from build123d import *

# Parameters (mm, degrees)
EXTRUDE_1_DEPTH     = 16
SKETCH_2_W          = 18.798290213
SKETCH_2_H          = 18.208539932
SKETCH_2_R          = 8
CUT_EXTRUDE_1_DEPTH = 16


with BuildPart() as part:
    # 草图1 → 凸台-拉伸1 (new body)
    with BuildSketch(Plane.XY):
        with BuildLine():
            Line((-8, 0), (-8, 16))
            Line((-8, 16), (8, 16))
            Line((8, 16), (8, 0))
            ThreePointArc((8, 0), (0, -8), (-8, 0))
        make_face()
    extrude(amount=EXTRUDE_1_DEPTH)

    # 草图2 → 切除-拉伸1 (cut)
    with BuildSketch(Plane(origin=(0, 16, 0), x_dir=(1, 0, 0), z_dir=(0, 1, 0))):
        with Locations((-0.294875141, -7.797273341)):
            Rectangle(SKETCH_2_W, SKETCH_2_H)
        with Locations((0, -8)):
            Circle(SKETCH_2_R, mode=Mode.SUBTRACT)
    extrude(amount=-CUT_EXTRUDE_1_DEPTH, mode=Mode.SUBTRACT)


solid = part.part
Geometry check sheet. Reference: the model listing, model coordinates, mm. A direction names the side the tool comes from. Round coordinates to 2 decimals unless told otherwise and drop trailing zeros. Loops run counter-clockwise (first coordinate to the right, second up) from the corner with the lowest first, then second, coordinate; pieces in that order, holes last.
Item 1: Cross-section at A-A on x = 1.5. Record the boundary of the cut face in (y, z), then the cut area to 3 significant figures.
Item 2: Cross-section at B-B on z = 15. Record the boundary of the cut face in (x, y), then the cut area to 3 significant figures.
Item 3: Thickness scan on line 1 (X direction, y = 11.25, z = 7.75); line 2 (X direction, y = -1, z = 14.5); line 3 (Y direction, x = -1.75, z = 10.5). Record the ranges inside material, lowest first.
Item 4: Gauge pin test, flat ends, axial feed: pin 1 (1.5 mm diameter, centred on y = 10.5, z = 5.5, fed in from +X); pin 2 (1 mm diameter, centred on x = -1, y = 2.5, fed in from +Z). Record the tip position at first contact, or that the pin passes through.
Item 5: Access from +Z, -Z, +X, -X, +Y, -Y to the whole of each face (thin tool, end or side, straight path). Record for faces 1 (the flat face through (6, 0, 14)), 2 (the flat face through (6, 0, 2)), 3 (the flat face through (-6, 0, 2)), 4 (the flat face through (-6, 0, 14)).
Item 6: Cross-section at C-C on y = -2.5. Record the boundary of the cut face in (x, z).
Item 7: Cross-section at D-D on x = -6.5. Record the boundary of the cut face in (y, z).
Answer sheet:
1. outline: (-7.86, 0) - (0, 0) - (0, 0.14) - (16, 0.14) - (16, 15.86) - (0, 15.86) - (0, 16) - (-7.86, 16) - close
1. area: 377 mm2
2. outline: (-8, 0) arc R8 ccw to (8, 0) - (3.87, 0) - (3.87, 16) - (-3.87, 16) - (-3.87, 0) - close
2. area: 224 mm2
3. line 1: x = -8 to 8
3. line 2: x = -7.94 to 7.94
3. line 3: y = -7.81 to 16
4. pin 1: stops at x = 7.81
4. pin 2: stops at z = 15.98
5. face 1: +Z, +X, +Y
5. face 2: -Z, +X, +Y
5. face 3: -Z, -X, +Y
5. face 4: +Z, -X, +Y
6. outline: (-7.6, 0) - (7.6, 0) - (7.6, 16) - (-7.6, 16) - close
7. outline: (-4.66, 0) - (0, 0) - (0, 3.34) - (16, 3.34) - (16, 12.66) - (0, 12.66) - (0, 16) - (-4.66, 16) - close
